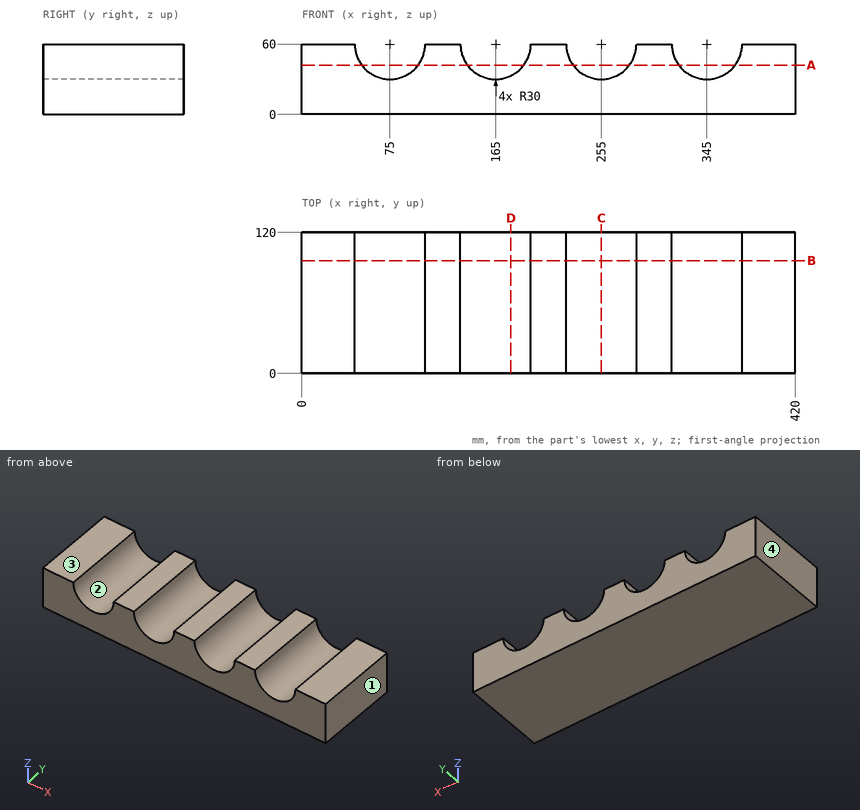
Could you check a few things on this drawing? It's one solid part, dimensions in mm from its lowest x, y, z. Round coordinates to 2 decimals unless told otherwise and drop trailing zeros. Loops run counter-clockwise (first coordinate to the right, second up) from the corner with the lowest first, then second, coordinate; pieces in that order, holes last. Notation, with made-up numbers: M 81.5,79.5 L 88.5,79.5 A5 ccw 88.5,83.5 Z; hole C 45.25,56 d5. An arc over 180 degrees is marked long. Write each question's results on one line, items separated by ' | '. Start each with the question number.
(1) Thinking about a two-plate mould opening in X: for the marked faces 1, 2, 3 and 4, which applies, pulls with the +X half, pulls with the -X half, needs draft (parallel to the pull), parting line crosses it, or undercut?
(2) I want a section at C-C (x = 255). Please give me the cut outline in (y, z).
(3) I want a section at A-A (z = 42). Please give me the cut outline in (x, y).
(4) I want a section at D-D (x = 178). Please give me the cut outline in (y, z), then the cut area to 3 significant figures.
(5) I want a section at B-B (y = 96). Please give me the cut outline in (x, z), then the cut area to 3 significant figures.
(6) If I drill on probe 1 along X at (y, z) = (77, 33); probe 2 along X at (y, z) = (102, 52); probe 3 along Z at (x, y) = (255, 85.5), over which ranges is the centre line in solid material (lowest first)? Write a range as from..to.
Solved:
1) face 1: pulls with the +X half | face 2: undercut | face 3: needs draft | face 4: pulls with the -X half
2) outline: M 0,0 L 120,0 L 120,30 L 0,30 Z
3) outline: M 0,0 L 51,0 L 51,120 L 0,120 Z; M 99,0 L 141,0 L 141,120 L 99,120 Z; M 189,0 L 231,0 L 231,120 L 189,120 Z; M 279,0 L 321,0 L 321,120 L 279,120 Z; M 369,0 L 420,0 L 420,120 L 369,120 Z
4) outline: M 0,0 L 120,0 L 120,32.96 L 0,32.96 Z | area: 3,960 mm²
5) outline: M 0,0 L 420,0 L 420,60 L 375,60 A30 cw 315,60 L 285,60 A30 cw 225,60 L 195,60 A30 cw 135,60 L 105,60 A30 cw 45,60 L 0,60 Z | area: 19,500 mm²
6) probe 1: x = 0..61.92, 88.08..151.92, 178.08..241.92, 268.08..331.92, 358.08..420 | probe 2: x = 0..46.09, 103.91..136.09, 193.91..226.09, 283.91..316.09, 373.91..420 | probe 3: z = 0..30
